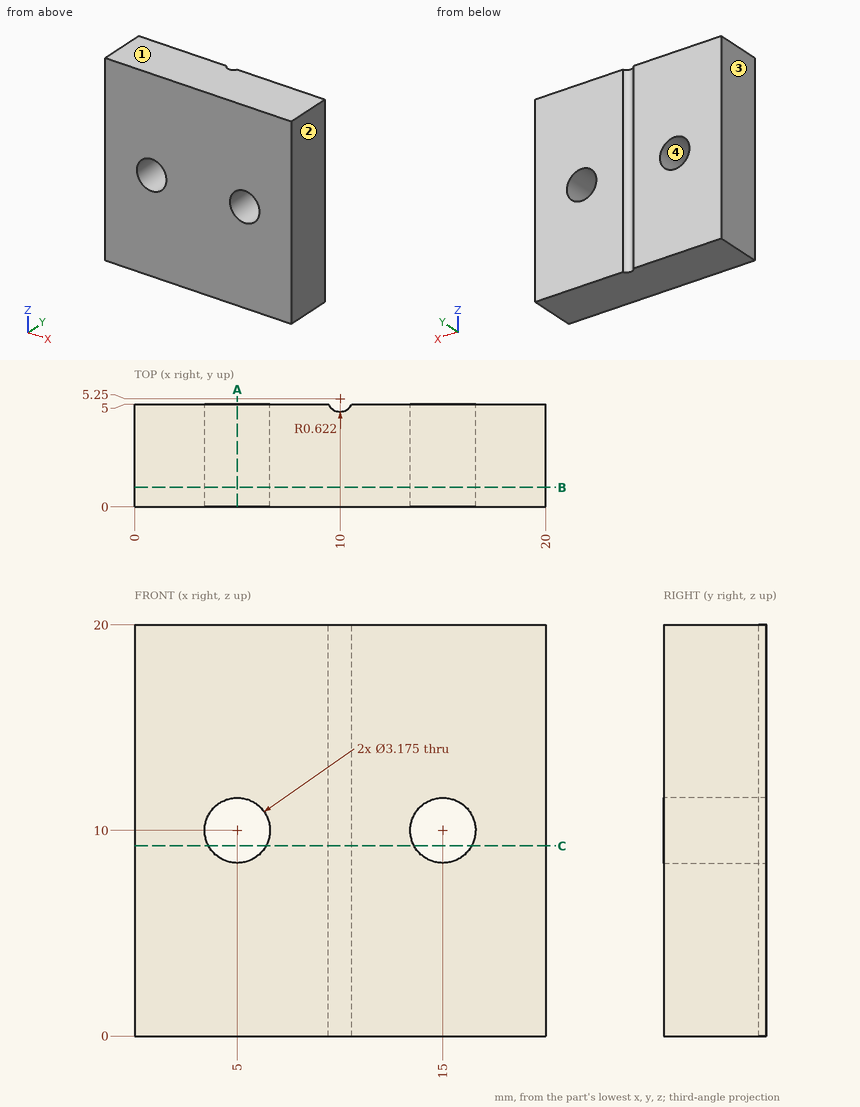
Could you check a few things on this drawing? It's one solid part, dimensions in mm from its lowest x, y, z. Give positions to 0.01 mm unless a question says otherwise; leave off trailing zeros. Write each loop counter-clockwise with the first axis right and the second up, starting at its lowest first coordinate (ties: lowest second). Pieces come first, ordered by that corner, then holes. Notation, with made-up numbers: M 58,78 L 82,78 A18 ccw 82,83 Z; hole C 2.5,36.25 d10. An arc over 180 degrees is marked long. Put each result on its own line as item: value. Start each with the question number.
Item 1: If we section it at C-C, the plane z = 9.25: Count the separate pieces of the cut face and the enclosed holes in it, then the cut area to 3 significant figures.
Item 2: If we section it at A-A, the plane x = 5: Write out the boundary of the cut face in (y, z).
Item 3: Will this pin go through, and if not, where does the flat tip stop? pin 1 (2 mm diameter, centred on x = 14, y = 2.5, fed in from -Z).
Item 4: I need wall thicknesses on L1, parallel to X at y = 3.75, z = 10; L2, parallel to X at y = 0.6, z = 9.5; L3, parallel to Z at x = 5.5, y = 1.05. Which ranges of each line are inside material? Lowest first, please. Write a range as from..to.
Item 5: Thinking about a two-plate mould opening in X: for the marked faces 1, 2, 3 and 4, which applies, +X half, -X half, draft (parallel to the pull), parting line (faces both ways), or undercut?
Item 6: If we section it at B-B, the plane y = 0.95: Write out the boundary of the cut face in (x, z) (1 decimal), then the cut area to 3 significant figures.
Values:
1. separate pieces: 3
1. enclosed holes: 0
1. area: 71.7 mm²
2. outline: M 0,0 L 5,0 L 5,8.41 L 0,8.41 Z; M 0,11.59 L 5,11.59 L 5,20 L 0,20 Z
3. pin 1: z = 0
4. L1: 0..3.41, 6.59..13.41, 16.59..20
4. L2: 0..3.49, 6.51..13.49, 16.51..20
4. L3: 0..8.49, 11.51..20
5. face 1: draft
5. face 2: +X half
5. face 3: -X half
5. face 4: undercut
6. outline: M 0,0 L 20,0 L 20,20 L 0,20 Z; hole C 5,10 d3.2; hole C 15,10 d3.2
6. area: 384 mm²
